from build123d import *

# Parameters (mm, degrees)
F1_DEPTH = 10


with BuildPart() as f1:
    # F0 (on Top) → F1 (new body)
    with BuildSketch(Plane.XY):
        with BuildLine():
            ThreePointArc((10.0000002235, 5.473572465), (11.0444556803, 2.8248891529), (11.4, 0))
            ThreePointArc((11.4, 0), (-2.8248896039, -11.0444555649), (-9.9999997765, 5.4735732817))
            Line((-9.9999997765, 5.4735732817), (-9.9999997765, 6.6332499177))
            ThreePointArc((-9.9999997765, 6.6332499177), (-3.4641018087, -11.4891252347), (12, 0))
            ThreePointArc((12, 0), (11.4891253514, 3.4641014216), (10.0000002235, 6.6332492437))
            Line((10.0000002235, 6.6332492437), (10.0000002235, 5.473572465))
        make_face()
        with BuildLine():
            ThreePointArc((-9.9999997765, 5.4735732817), (4.655e-07, 11.4), (10.0000002235, 5.473572465))
            Line((10.0000002235, 5.473572465), (10.0000002235, 6.6332492437))
            ThreePointArc((10.0000002235, 6.6332492437), (4.044e-07, 12), (-9.9999997765, 6.6332499177))
            Line((-9.9999997765, 6.6332499177), (-9.9999997765, 5.4735732817))
        make_face()
        with BuildLine():
            ThreePointArc((-9.9999997765, 6.6332499177), (4.044e-07, 12), (10.0000002235, 6.6332492437))
            Line((10.0000002235, 6.6332492437), (10.0000002235, 20))
            Line((10.0000002235, 20), (-9.9999997765, 20))
            Line((-9.9999997765, 20), (-9.9999997765, 6.6332499177))
        make_face()
    extrude(amount=F1_DEPTH)


solid = f1.part
Input: part model. Units: mm. Frame: model coordinates. A direction names the side the tool comes from. Round coordinates to 2 decimals unless told otherwise and drop trailing zeros. Write each loop counter-clockwise with the first axis right and the second up, starting at its lowest first coordinate (ties: lowest second). Pieces come first, ordered by that corner, then holes.
1) Contact query for flat-ended pins moving along their axis: P1, Ø8, axis at x = -2.5, y = 6.5, coming from the -Z side; P2, Ø6, axis at y = 5, z = 6, coming from the -X side; P3, Ø4, axis at x = -7, z = 3, coming from the -Y side. Output: stop coordinate, or through.
2) Ray query, L1, parallel to X at y = 0, z = 3.75; L2, parallel to Y at x = 5.25, z = 3.5; L3, parallel to X at y = -6, z = 0.5. Return the intervals inside material, ascending.
3) Reachability of faces 1 (the flat face through (-10, 13, 5)), 2 (the flat face through (0, 20, 5)), 3 (the flat face through (10, 13, 5)) from +Z, -Z, +X, -X, +Y, -Y: full face, straight path, thin tool, end or side. Return the list, or none.
4) Cut plane D-D (y = 17). Return the cut outline in (x, z), then the cut area to 3 significant figures.
5) Cut plane C-C (z = 1.5). Return the cut outline in (x, y), then the cut area to 3 significant figures.
6) Cut plane B-B (y = 1.5). Return the cut outline in (x, z), then the cut area to 3 significant figures.
7) Cut plane A-A (x = 0). Return the cut outline in (y, z), then the cut area to 3 significant figures.
Geometry says:
1. P1: passes through
1. P2: stops at x = -11.83
1. P3: stops at y = -10.91
2. L1: x = -12 to -11.4, 11.4 to 12
2. L2: y = -10.79 to -10.12, 10.12 to 20
2. L3: x = -10.39 to -9.69, 9.69 to 10.39
3. face 1: +Z, -Z, -X, +Y
3. face 2: +Z, -Z, +X, -X, +Y
3. face 3: +Z, -Z, +X, +Y
4. outline: (-10, 0) - (10, 0) - (10, 10) - (-10, 10) - close
4. area: 200 mm2
5. outline: (-10, 6.63) arc R12 ccw (long way) to (10, 6.63) - (10, 20) - (-10, 20) - close; hole circle Ø22.8 at (0, 0)
5. area: 236 mm2
6. outline: (-11.91, 0) - (-11.3, 0) - (-11.3, 10) - (-11.91, 10) - close; (11.3, 0) - (11.91, 0) - (11.91, 10) - (11.3, 10) - close
6. area: 12.1 mm2
7. outline: (-12, 0) - (-11.4, 0) - (-11.4, 10) - (-12, 10) - close; (11.4, 0) - (20, 0) - (20, 10) - (11.4, 10) - close
7. area: 92.0 mm2
